Source: CAD feature listing. Evaluate the final solid. Frame: model axes, mm. Face numbers are marked on the shaded views. A direction names the side the tool comes from. Round coordinates to 2 decimals unless told otherwise and drop trailing zeros. Order: outer loops, then holes, each group sorted by start corner. A loop starts at its lowest first (then second) coordinate and runs counter-clockwise, first axis right, second up.
Autodesk Inventor part; units mm, degrees
ref_plane "Work Plane1" through (0, 0, 1.25) normal (0, 0, 1) x (1, 0, 0)
ref_plane "YZ Plane" through (0, 0, 0) normal (1, 0, 0) x (0, 1, 0)
ref_plane "XZ Plane" through (0, 0, 0) normal (0, 1, 0) x (-1, 0, 0)
sketch "Sketch1" plane through (0, 0, 0) normal (0, 0, 1) x (1, 0, 0)
  circle A0 centre (0, 0) radius 3
  dimension "d0" = 6
extrude "Extrusion1" add sketch "Sketch1" along normal blind 2.5
hole "Hole1" at (0, 0, 2.5) direction (0, 0, -1) diameter 3 end through all
sketch "Sketch2" plane through (0, 0, 2.5) normal (0, 0, 1) x (1, 0, 0)
  circle A0 centre (0, 0) radius 2.5
  circle A1 centre (0, 0) radius 2
  dimension "d12" = 5
  dimension "d13" = 4
extrude "Extrusion2" cut sketch "Sketch2" against normal blind 0.5
ref_plane "Work Plane1" through (0, 0, 1.25) normal (0, 0, 1) x (1, 0, 0)
mirror "Mirror1" about plane through (0, 0, 1.25) normal (0, 0, 1) of "Extrusion2"
properties part number "bearing_3x6x2,5" material "Stainless Steel"
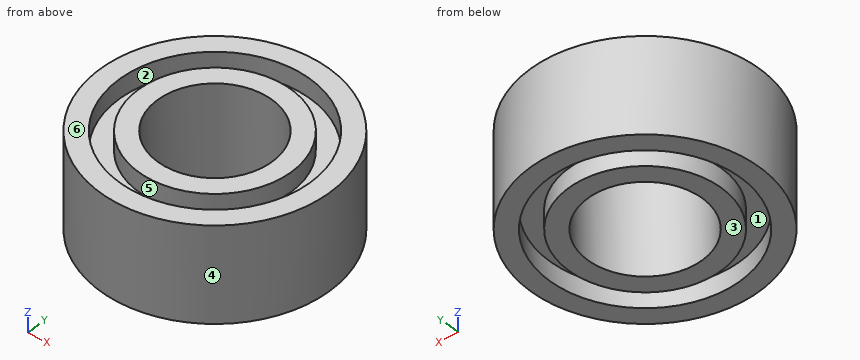
1. Line query: line 1 along Y through (x, z) = (0, 0.2); line 2 along Y through (x, z) = (0, 1.5); line 3 along X through (y, z) = (-0.45, 0.4). Output: solid intervals per line, ascending.
2. Section A-A on y = 0. Return loops of the section in (x, z), plus the area to 3 significant figures.
3. Access query for the marked faces 1, 2 and 3. Directions: +Z, -Z, +X, -X, +Y, -Y. A direction counts if a zero-diameter tool reaches every point of the face in a straight line with its end or side. Return the directions, or none.
4. Section D-D on x = -2.35. Return loops of the section in (y, z), plus the area to 3 significant figures.
5. First-contact query: pin 1 (1 mm diameter, centred on x = -1.5, y = 2, fed in from -Z). Flat tip, straight axial feed; report the tip coordinate or a pass-through.
6. Pull-direction query (X, two-part tool) for the marked faces 4, 5 and 6; classes: released by +X, released by -X, zero draft, split by the parting line, or undercut.
7. Section C-C on z = 1.75. Return loops of the section in (x, y).
Result:
1. line 1: y = -3 to -2.5, -2 to -1.5, 1.5 to 2, 2.5 to 3
1. line 2: y = -3 to -1.5, 1.5 to 3
1. line 3: x = -2.97 to -2.46, -1.95 to -1.43, 1.43 to 1.95, 2.46 to 2.97
2. outline: (-3, 0) - (-2.5, 0) - (-2.5, 0.5) - (-2, 0.5) - (-2, 0) - (-1.5, 0) - (-1.5, 2.5) - (-2, 2.5) - (-2, 2) - (-2.5, 2) - (-2.5, 2.5) - (-3, 2.5) - close; (1.5, 0) - (2, 0) - (2, 0.5) - (2.5, 0.5) - (2.5, 0) - (3, 0) - (3, 2.5) - (2.5, 2.5) - (2.5, 2) - (2, 2) - (2, 2.5) - (1.5, 2.5) - close
2. area: 6.50 mm2
3. face 1: -Z
3. face 2: +Z
3. face 3: -Z, +X, -X, +Y, -Y
4. outline: (-1.86, 0) - (-0.85, 0) - (-0.85, 0.5) - (0.85, 0.5) - (0.85, 0) - (1.86, 0) - (1.86, 2.5) - (0.85, 2.5) - (0.85, 2) - (-0.85, 2) - (-0.85, 2.5) - (-1.86, 2.5) - close
4. area: 7.62 mm2
5. pin 1: stops at z = 0
6. face 4: split by the parting line
6. face 5: undercut
6. face 6: zero draft
7. outline: circle Ø6 at (0, 0); hole circle Ø3 at (0, 0)
